from build123d import *

# Parameters (mm, degrees)
SKETCH3_R           = 1.5
BOSS_EXTRUDE1_DEPTH = 3
BOSS_EXTRUDE2_DEPTH = 3
SKETCH5_R           = 1.5
CUT_EXTRUDE1_DEPTH  = 3


with BuildPart() as part:
    # Sketch3 → Boss-Extrude1 (new body)
    # profile 1 of 2: a face of its own
    with BuildSketch(Plane(origin=(0, 0, 0), x_dir=(1, 0, 0), z_dir=(0, 1, 0))):
        with BuildLine():
            Line((-6, 5), (6, 5))
            ThreePointArc((6, 5), (7.414213562, 4.414213562), (8, 3))
            Line((8, 3), (8, 0))
            Line((8, 0), (-8, 0))
            Line((-8, 0), (-8, 3))
            ThreePointArc((-8, 3), (-7.414213562, 4.414213562), (-6, 5))
        make_face()
    # profile 2 of 2: a face of its own
    with BuildSketch(Plane(origin=(0, 0, 0), x_dir=(1, 0, 0), z_dir=(0, 1, 0))):
        with BuildLine():
            Line((-5.5, 0), (5.5, 0))
            Line((5.5, 0), (5.5, -25.5))
            ThreePointArc((5.5, -25.5), (4.914213562, -26.914213562), (3.5, -27.5))
            Line((3.5, -27.5), (-3.5, -27.5))
            ThreePointArc((-3.5, -27.5), (-4.914213562, -26.914213562), (-5.5, -25.5))
            Line((-5.5, -25.5), (-5.5, 0))
        make_face()
        with Locations(Location((0, -5.5, 0), (0, 0, 270))):
            Circle(SKETCH3_R, mode=Mode.SUBTRACT)
        with Locations(Location((0, -23, 0), (0, 0, 270))):
            Circle(SKETCH3_R, mode=Mode.SUBTRACT)
    extrude(amount=BOSS_EXTRUDE1_DEPTH)

    # Sketch4 → Boss-Extrude2 (add)
    with BuildSketch(Plane(origin=(0, 3, 0), x_dir=(1, 0, 0), z_dir=(0, 1, 0))):
        with BuildLine():
            Line((-8, 0), (8, 0))
            Line((8, 0), (8, 11))
            ThreePointArc((8, 11), (6.535533906, 14.535533906), (3, 16))
            Line((3, 16), (-3, 16))
            ThreePointArc((-3, 16), (-6.535533906, 14.535533906), (-8, 11))
            Line((-8, 11), (-8, 0))
        make_face()
    extrude(amount=-BOSS_EXTRUDE2_DEPTH)

    # Sketch5 → Cut-Extrude1 (cut)
    with BuildSketch(Plane(origin=(0, 0, 0), x_dir=(-1, 0, 0), z_dir=(0, -1, 0))):
        with Locations(Location((0, 10, 0), (0, 0, 90))):
            Circle(SKETCH5_R)
    extrude(amount=-CUT_EXTRUDE1_DEPTH, mode=Mode.SUBTRACT)


solid = part.part
Geometry check sheet. Reference: the model listing, model coordinates, mm. A direction names the side the tool comes from. Coordinates: 2 decimals unless noted, no trailing zeros. Order: outer loops, then holes, each group sorted by start corner. A loop starts at its lowest first (then second) coordinate and runs counter-clockwise, first axis right, second up. Notation, with made-up numbers: (-32.75, 48) - (2.25, 48) arc R20 ccw to (2.25, 73) - close; hole circle Ø2 at (-19.5, -22). An arc over 180 degrees is marked (long way). Answer in a Markdown table with one row per item. Add a question column.
1) Gauge pin test, flat end, axial feed: P1, Ø0.8, axis at x = -6.5, y = 1.5, coming from the +Z side. Record the tip position at first contact, or that the pin passes through.
2) Set-up check for faces 1 (the flat face through (-2, 0, 5)), 2 (the flat face through (7, 1, 0)), 3 (the flat face through (-5.5, 1, 13)): record each of +Z, -Z, +X, -X, +Y, -Y from which the full face is reachable in a straight line by a thin tool's end or side.
3) Cross-section at D-D, the plane z = -10. Record the cut outline in (x, y), then the cut area to 3 significant figures.
4) Material ranges on line 1 along Z through (x, y) = (-1, 1.65); line 2 along X through (y, z) = (1.55, 5.5); line 3 along X through (y, z) = (2, -10), recorded low to high. Write a range as [from, to].
5) Release check for a two-part mould opening along Z. For faces 4 (the cylindrical face through (0.07, 1.48, -8.5)), 5 (the flat face through (5.5, 1, 13)), 6 (the flat face through (-7, 1, 0)) record: +Z half, -Z half, draft (parallel to the pull), parting line (faces both ways), or undercut.
6) Cross-section at A-A, the plane z = 5.5. Record the cut outline in (x, y).
7) Cross-section at C-C, the plane y = 1.6. Record the cut outline in (x, z), then the cut area to 3 significant figures.
8) Cross-section at B-B, the plane x = 0. Record the cut outline in (y, z).
Check result:
| question | item | result |
|---|---|---|
| 1 | P1 | stops at z = 0 |
| 2 | face 1 | +Z, -Z, +X, -X, -Y |
| 2 | face 2 | +Z, +X, +Y, -Y |
| 2 | face 3 | +Z, -X, +Y, -Y |
| 3 | outline | (-8, 0) - (-1.5, 0) - (-1.5, 3) - (-8, 3) - close; (1.5, 0) - (8, 0) - (8, 3) - (1.5, 3) - close |
| 3 | area | 39.0 mm² |
| 4 | line 1 | z = [-16, -11.12], [-8.88, 4.38], [6.62, 21.88], [24.12, 27.5] |
| 4 | line 2 | x = [-5.5, -1.5], [1.5, 5.5] |
| 4 | line 3 | x = [-8, -1.5], [1.5, 8] |
| 5 | face 4 | undercut |
| 5 | face 5 | draft |
| 5 | face 6 | +Z half |
| 6 | outline | (-5.5, 0) - (-1.5, 0) - (-1.5, 3) - (-5.5, 3) - close; (1.5, 0) - (5.5, 0) - (5.5, 3) - (1.5, 3) - close |
| 7 | outline | (-8, -11) arc R5 ccw to (-3, -16) - (3, -16) arc R5 ccw to (8, -11) - (8, 0) - (5.5, 0) - (5.5, 25.5) arc R2 ccw to (3.5, 27.5) - (-3.5, 27.5) arc R2 ccw to (-5.5, 25.5) - (-5.5, 0) - (-8, 0) - close; hole circle Ø3 at (0, -10); hole circle Ø3 at (0, 5.5); hole circle Ø3 at (0, 23) |
| 7 | area | 525 mm² |
| 8 | outline | (0, -16) - (3, -16) - (3, -11.5) - (0, -11.5) - close; (0, -8.5) - (3, -8.5) - (3, 4) - (0, 4) - close; (0, 7) - (3, 7) - (3, 21.5) - (0, 21.5) - close; (0, 24.5) - (3, 24.5) - (3, 27.5) - (0, 27.5) - close |
